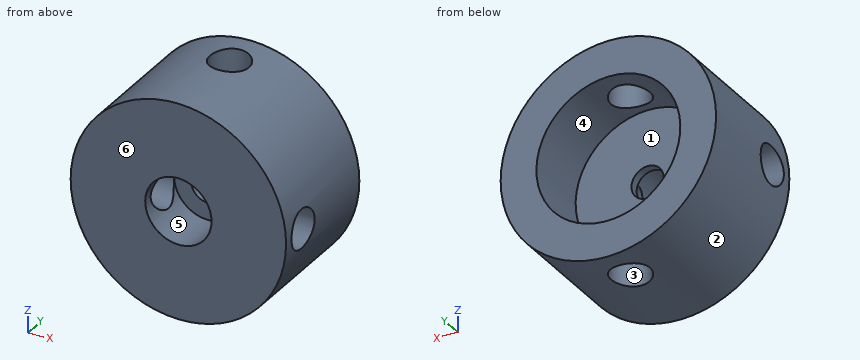
```python
from build123d import *

# Parameters (mm, degrees)
SKETCH1_R           = 9.525
SKETCH1_R_2         = 2.9337
BOSS_EXTRUDE1_DEPTH = 5.08
SKETCH2_R           = 9.525
SKETCH2_R_2         = 6.3627
BOSS_EXTRUDE2_DEPTH = 5.842
SKETCH3_R           = 1.7272
CUT_EXTRUDE1_DEPTH  = 12.7
SKETCH4_R           = 1.7272
CUT_EXTRUDE2_DEPTH  = 12.7
SKETCH6_R           = 4.231677678
SKETCH6_R_2         = 1.4224
BOSS_EXTRUDE4_DEPTH = 0.762


with BuildPart() as part:
    # Sketch1 → Boss-Extrude1 (new body)
    with BuildSketch(Plane(origin=(0, 0, 0), x_dir=(1, 0, 0), z_dir=(0, 1, 0))):
        with Locations(Location((0, 0, 0), (0, 0, 270))):
            Circle(SKETCH1_R)
        with Locations(Location((0, 0, 0), (0, 0, 270))):
            Circle(SKETCH1_R_2, mode=Mode.SUBTRACT)
    extrude(amount=BOSS_EXTRUDE1_DEPTH)

    # Sketch2 → Boss-Extrude2 (add)
    with BuildSketch(Plane(origin=(0, 5.08, 0), x_dir=(1, 0, 0), z_dir=(0, 1, 0))):
        with Locations(Location((0, 0, 0), (0, 0, 270))):
            Circle(SKETCH2_R)
        with Locations(Location((0, 0, 0), (0, 0, 270))):
            Circle(SKETCH2_R_2, mode=Mode.SUBTRACT)
    extrude(amount=BOSS_EXTRUDE2_DEPTH)

    # Sketch3 → Cut-Extrude1 (cut, symmetric)
    with BuildSketch(Plane.XY):
        with Locations((0, 7.62)):
            Circle(SKETCH3_R)
    extrude(amount=CUT_EXTRUDE1_DEPTH, both=True, mode=Mode.SUBTRACT)

    # Sketch4 → Cut-Extrude2 (cut, symmetric)
    with BuildSketch(Plane(origin=(0, 0, 0), x_dir=(0, 0, -1), z_dir=(1, 0, 0))):
        with Locations((0, 2.54)):
            Circle(SKETCH4_R)
    extrude(amount=CUT_EXTRUDE2_DEPTH, both=True, mode=Mode.SUBTRACT)

    # Sketch6 → Boss-Extrude4 (add)
    with BuildSketch(Plane(origin=(0, 5.08, 0), x_dir=(1, 0, 0), z_dir=(0, 1, 0))):
        Circle(SKETCH6_R)
        with Locations(Location((0, 0, 0), (0, 0, 270))):
            Circle(SKETCH6_R_2, mode=Mode.SUBTRACT)
    extrude(amount=-BOSS_EXTRUDE4_DEPTH)


solid = part.part
```
Here's how the part is built. I have some questions about the finished solid (model axes, mm). Face numbers are marked on the shaded views. A direction names the side the tool comes from. Give positions to 0.01 mm unless a question says otherwise; leave off trailing zeros. Write each loop counter-clockwise with the first axis right and the second up, starting at its lowest first coordinate (ties: lowest second). Pieces come first, ordered by that corner, then holes. Notation, with made-up numbers: (18.25, 54.25) -> (49.25, 54.25) arc R18 ccw to (49.25, 71.25) -> close; hole circle Ø5 at (-3.5, 11). An arc over 180 degrees is marked (long way). Write each question's results on one line, items separated by ' | '.
Item 1: Suppose I cut it at B-B on y = 2.54. Write out the boundary of the cut face in (x, z) (3 decimals), plus the area to 3 significant figures.
Output:
outline: (-9.367, -1.727) arc R9.525 ccw to (9.367, -1.727) -> (2.371, -1.727) arc R2.934 cw to (-2.371, -1.727) -> close; (-9.367, 1.727) -> (-2.371, 1.727) arc R2.934 cw to (2.371, 1.727) -> (9.367, 1.727) arc R9.525 ccw to start | area: 212 mm^2
Item 2: Suppose I cut it at D-D on x = -5.25. Write out the boundary of the cut face in (y, z).
Output:
outline: (0, -7.95) -> (10.92, -7.95) -> (10.92, -3.59) -> (5.08, -3.59) -> (5.08, 3.59) -> (10.92, 3.59) -> (10.92, 7.95) -> (0, 7.95) -> close; hole circle Ø3.45 at (2.54, 0)
Item 3: Suppose I cut it at C-C on x = -0.5. Write out the boundary of the cut face in (y, z), plus the area to 3 significant figures.
Output:
outline: (0, -9.51) -> (5.97, -9.51) -> (5.97, -6.34) -> (5.08, -6.34) -> (5.08, -1.33) -> (4.32, -1.33) -> (4.32, -2.89) -> (0, -2.89) -> close; (0, 2.89) -> (4.32, 2.89) -> (4.32, 1.33) -> (5.08, 1.33) -> (5.08, 6.34) -> (5.97, 6.34) -> (5.97, 9.51) -> (0, 9.51) -> close; (9.27, -9.51) -> (10.92, -9.51) -> (10.92, -6.34) -> (9.27, -6.34) -> close; (9.27, 6.34) -> (10.92, 6.34) -> (10.92, 9.51) -> (9.27, 9.51) -> close | area: 85.7 mm^2
Item 4: On a 3-axis mill with a long thin cutter (end or side, diameter ignored), from which of +Z, -Z, +X, -X, +Y, -Y can I reach the whole of each face in a straight line? I mean the marked faces 4, 5 and 6. Say none if no direction works.
Output:
face 4: +Y | face 5: -Y | face 6: +Z, -Z, +X, -X, -Y
Item 5: For pin 1 Ø2 at (y, z) = (5, 4.5) entering from -X; pin 2 Ø3 at (x, y) = (1.5, 7) entering from -Z; pin 3 Ø4 at (x, y) = (-7, 3) entering from +Z; pin 4 Ø1.7 at (x, z) = (0, 0) entering from -Y, each with a flat end and sliding along its axis, tell me the tip position at first contact or that it passes through.
Output:
pin 1: stops at x = -8.86 | pin 2: stops at z = -9.52 | pin 3: stops at z = 8.11 | pin 4: passes through
Item 6: Suppose I cut it at A-A on z = 0. Write out the boundary of the cut face in (x, y) (3 decimals).
Output:
outline: (-9.525, 0) -> (-2.934, 0) -> (-2.934, 0.813) -> (-9.525, 0.813) -> close; (-9.525, 4.267) -> (-2.934, 4.267) -> (-2.934, 4.318) -> (-1.422, 4.318) -> (-1.422, 5.08) -> (-6.363, 5.08) -> (-6.363, 10.922) -> (-9.525, 10.922) -> close; (1.422, 4.318) -> (2.934, 4.318) -> (2.934, 4.267) -> (9.525, 4.267) -> (9.525, 10.922) -> (6.363, 10.922) -> (6.363, 5.08) -> (1.422, 5.08) -> close; (2.934, 0) -> (9.525, 0) -> (9.525, 0.813) -> (2.934, 0.813) -> close
Item 7: We'd pull the mould along Z, two halves only. Please class the marked faces 1, 2 and 3: pulls with the +Z half, pulls with the -Z half, needs draft (parallel to the pull), parting line crosses it, or undercut.
Output:
face 1: undercut | face 2: parting line crosses it | face 3: needs draft
Item 8: If I drill on L1, parallel to X at y = 4.95, z = 0 (3 decimals); L2, parallel to Y at x = 0, z = 6.5; L3, parallel to X at y = 8.5, z = 0 (3 decimals), over which ranges is the centre line in solid material (lowest first)?
Output:
L1: x = -9.525 to -1.422, 1.422 to 9.525 | L2: y = 0 to 5.89, 9.35 to 10.92 | L3: x = -9.525 to -6.363, 6.363 to 9.525
